```python
from build123d import *

# Parameters (mm, degrees)
SKETCH_1_W          = 15
SKETCH_1_H          = 15
SKETCH_1_W_2        = 12
SKETCH_1_H_2        = 12
EXTRUDE_1_DEPTH     = 135
SKETCH_2_R          = 2.7
CUT_EXTRUDE_1_DEPTH = 25
SKETCH_3_R          = 2.7
CUT_EXTRUDE_2_DEPTH = 25
SKETCH_4_R          = 5
CUT_EXTRUDE_3_DEPTH = 10
SKETCH_5_R          = 5
CUT_EXTRUDE_4_DEPTH = 10


with BuildPart() as part:
    # ｽｹｯﾁ1 → ﾎﾞｽ - 押し出し1 (new body)
    with BuildSketch(Plane.XY):
        Rectangle(SKETCH_1_W, SKETCH_1_H)
        Rectangle(SKETCH_1_W_2, SKETCH_1_H_2, mode=Mode.SUBTRACT)
    extrude(amount=EXTRUDE_1_DEPTH)

    # ｽｹｯﾁ2 → ｶｯﾄ - 押し出し1 (cut)
    with BuildSketch(Plane(origin=(7.5, 0, 0), x_dir=(0, 0, -1), z_dir=(1, 0, 0))):
        with Locations((-112.5, 0)):
            Circle(SKETCH_2_R)
        with Locations((-22.5, 0)):
            Circle(SKETCH_2_R)
    extrude(amount=-CUT_EXTRUDE_1_DEPTH, mode=Mode.SUBTRACT)

    # ｽｹｯﾁ3 → ｶｯﾄ - 押し出し2 (cut)
    with BuildSketch(Plane(origin=(0, 7.5, 0), x_dir=(1, 0, 0), z_dir=(0, 1, 0))):
        with Locations((0, -7.5)):
            Circle(SKETCH_3_R)
        with Locations((0, -127.5)):
            Circle(SKETCH_3_R)
    extrude(amount=-CUT_EXTRUDE_2_DEPTH, mode=Mode.SUBTRACT)

    # ｽｹｯﾁ4 → ｶｯﾄ - 押し出し3 (cut)
    with BuildSketch(Plane(origin=(0, 7.5, 0), x_dir=(1, 0, 0), z_dir=(0, 1, 0))):
        with Locations((0, -127.5)):
            Circle(SKETCH_4_R)
        with Locations((0, -7.5)):
            Circle(SKETCH_4_R)
    extrude(amount=-CUT_EXTRUDE_3_DEPTH, mode=Mode.SUBTRACT)

    # ｽｹｯﾁ5 → ｶｯﾄ - 押し出し4 (cut)
    with BuildSketch(Plane(origin=(7.5, 0, 0), x_dir=(0, 0, -1), z_dir=(1, 0, 0))):
        with Locations((-22.5, 0)):
            Circle(SKETCH_5_R)
        with Locations((-112.5, 0)):
            Circle(SKETCH_5_R)
    extrude(amount=-CUT_EXTRUDE_4_DEPTH, mode=Mode.SUBTRACT)


solid = part.part
```
Work out the finished part from the listing and answer in its coordinate system (mm). A direction names the side the tool comes from. Coordinates: 2 decimals unless noted, no trailing zeros. Loops run counter-clockwise (first coordinate to the right, second up) from the corner with the lowest first, then second, coordinate; pieces in that order, holes last. Notation, with made-up numbers: M 84.25,-3.75 L 126.25,-3.75 A22 cw 126.25,10.25 Z; hole C 74,-13 d9. An arc over 180 degrees is marked long. Use CSV: the item, a comma, the result in double quotes. Start each with the question number.
(1) For faces 5 (the face through (6, 0, 67)), 6 (the face through (6.76, 0.22, 27.495)), 7 (the face through (2.307, 6.76, 131.936)), determine the directions among +Z, -Z, +X, -X, +Y, -Y from which every point of the face is accessible in a straight line to the end or side of a thin tool.
(2) Given pin 1 Ø3 at (y, z) = (0, 112.5) entering from +X, flat-ended and moving along its own axis, determine where the tip first touches the part or whether it passes through.
(3) Find section C-C, the plane z = 54. Give the vertices of the cut face in (x, y), then the cut area to 3 significant figures.
(4) Find section B-B, the plane y = 0. Give the vertices of the cut face in (x, z).
(5) Find section A-A, the plane z = 127.5. Give the vertices of the cut face in (x, y).
(6) Consider line 1 (Z direction, x = 0, y = 6.45); line 2 (Z direction, x = 0, y = -7.05); line 3 (Y direction, x = 3, z = 93). Determine where each line is inside the solid, lowest interval first.
(7) Find section D-D, the plane x = 0.25. Give the vertices of the cut face in (y, z), then the cut area to 3 significant figures.
(8) For a pull along Z with two mould halves and no side action, classify faces 1 (the face through (1.246, -6.74, 129.895)), 2 (the face through (-6.74, -1.034, 20.006)), 3 (the face through (7.5, 0, 67)), 4 (the face through (-7, 0, 0)) as +Z half, -Z half, draft (parallel to the pull), parting line (faces both ways), or undercut.
Recorded:
1,face 5,"+Z, -Z"
1,face 6,"+X"
1,face 7,"+Y"
2,pin 1,"passes through"
3,outline,"M -7.5,-7.5 L 7.5,-7.5 L 7.5,7.5 L -7.5,7.5 Z; hole M -6,-6 L 6,-6 L 6,6 L -6,6 Z"
3,area,"81.0 mm^2"
4,outline,"M -7.5,0 L -6,0 L -6,19.8 L -7.5,19.8 Z; M -7.5,25.2 L -6,25.2 L -6,109.8 L -7.5,109.8 Z; M -7.5,115.2 L -6,115.2 L -6,135 L -7.5,135 Z; M 6,0 L 7.5,0 L 7.5,17.5 L 6,17.5 Z; M 6,27.5 L 7.5,27.5 L 7.5,107.5 L 6,107.5 Z; M 6,117.5 L 7.5,117.5 L 7.5,135 L 6,135 Z"
5,outline,"M -7.5,-7.5 L -2.7,-7.5 L -2.7,-6 L -6,-6 L -6,6 L -5,6 L -5,7.5 L -7.5,7.5 Z; M 2.7,-7.5 L 7.5,-7.5 L 7.5,7.5 L 5,7.5 L 5,6 L 6,6 L 6,-6 L 2.7,-6 Z"
6,line 1,"z = 0 to 2.5, 12.5 to 122.5, 132.5 to 135"
6,line 2,"z = 0 to 4.8, 10.2 to 124.8, 130.2 to 135"
6,line 3,"y = -7.5 to -6, 6 to 7.5"
7,outline,"M -7.5,0 L -6,0 L -6,4.81 L -7.5,4.81 Z; M -7.5,10.19 L -6,10.19 L -6,124.81 L -7.5,124.81 Z; M -7.5,130.19 L -6,130.19 L -6,135 L -7.5,135 Z; M 6,0 L 7.5,0 L 7.5,2.51 L 6,2.51 Z; M 6,12.49 L 7.5,12.49 L 7.5,122.51 L 6,122.51 Z; M 6,132.49 L 7.5,132.49 L 7.5,135 L 6,135 Z"
7,area,"359 mm^2"
8,face 1,"undercut"
8,face 2,"undercut"
8,face 3,"draft"
8,face 4,"-Z half"
